CAD build for the part. Positions are in the model's coordinates, mm. Face numbers are marked on the shaded views. Coordinates: 2 decimals unless noted, no trailing zeros. Write each loop counter-clockwise with the first axis right and the second up, starting at its lowest first coordinate (ties: lowest second). Pieces come first, ordered by that corner, then holes. Notation, with made-up numbers: M -27.75,59 L -12.75,59 A26 cw -12.75,75 Z; hole C 63,55.5 d10. An arc over 180 degrees is marked long. Answer as CSV lines item,"result". Start each with the question number.
```python
from build123d import *

# Parameters (mm, degrees)
SKETCH_1_R      = 8.5
SKETCH_1_R_2    = 2.1
EXTRUDE_1_DEPTH = 6
FILLET_1_R      = 15
FILLET_2_R      = 2
SKETCH_2_R      = 2.1
EXTRUDE_2_DEPTH = 5
SKETCH_3_W      = 10
SKETCH_3_H      = 30
SKETCH_3_R      = 2.1
EXTRUDE_3_DEPTH = 7
FILLET_4_R      = 2
FILLET_5_R      = 2
CHAMFER_1_SIZE  = 1


with BuildPart() as part:
    # 草图1 → 凸台-拉伸1 (new body)
    with BuildSketch(Plane(origin=(0, 0, 0), x_dir=(1, 0, 0), z_dir=(0, 1, 0))):
        Polygon((0, 0), (100, 0), (129.781745931, -29.781745931), (158.066017178, -1.497474683), (132.13708499, 24.431457505), (70, 24.431457505), (30, 24.431457505), (-32.13708499, 24.431457505), (-58.066017178, -1.497474683), (-29.781745931, -29.781745931), align=None)
        with Locations(Location((-30.5, -5, 0), (0, 0, 270))):
            Circle(SKETCH_1_R, mode=Mode.SUBTRACT)
        with Locations(Location((130.5, -5, 0), (0, 0, 270))):
            Circle(SKETCH_1_R, mode=Mode.SUBTRACT)
        with Locations(Location((0, 10, 0), (0, 0, 270))):
            Circle(SKETCH_1_R_2, mode=Mode.SUBTRACT)
        with Locations(Location((100, 10, 0), (0, 0, 270))):
            Circle(SKETCH_1_R_2, mode=Mode.SUBTRACT)
    extrude(amount=EXTRUDE_1_DEPTH)

    # 圆角1
    fillet_1_edges = [part.edges().sort_by_distance(p)[0] for p in [
        (-29.781745931, 3, 29.781745931),
        (-58.066017178, 3, 1.497474683),
        (158.066017178, 3, 1.497474683),
        (129.781745931, 3, 29.781745931),
    ]]
    fillet(fillet_1_edges, radius=FILLET_1_R)

    # 圆角2
    fillet_2_edges = [part.edges().sort_by_distance(p)[0] for p in [
        (100, 3, 0),
        (0, 3, 0),
    ]]
    fillet(fillet_2_edges, radius=FILLET_2_R)

    # 草图2 → 凸台-拉伸2 (add)
    # profile 1 of 4: a face of its own
    with BuildSketch(Plane.XY):
        Polygon((17, 6), (23, 6), (27, 6), (27, 30), (17, 30), align=None)
        with Locations((23, 15)):
            Circle(SKETCH_2_R, mode=Mode.SUBTRACT)
        with Locations((23, 25)):
            Circle(SKETCH_2_R, mode=Mode.SUBTRACT)
    # profile 2 of 4: a face of its own
    with BuildSketch(Plane.XY):
        Polygon((27, 6), (23, 6), (17, 6), (17, 0), (27, 0), align=None)
    # profile 3 of 4: a face of its own
    with BuildSketch(Plane.XY):
        Polygon((68, 30), (68, 6), (72, 6), (78, 6), (78, 30), align=None)
        with Locations((72, 15)):
            Circle(SKETCH_2_R, mode=Mode.SUBTRACT)
        with Locations((72, 25)):
            Circle(SKETCH_2_R, mode=Mode.SUBTRACT)
    # profile 4 of 4: a face of its own
    with BuildSketch(Plane.XY):
        Polygon((72, 6), (68, 6), (68, 0), (78, 0), (78, 6), align=None)
    extrude(amount=-EXTRUDE_2_DEPTH)

    # 草图3 → 凸台-拉伸3 (add)
    # profile 1 of 2: a face of its own
    with BuildSketch(Plane(origin=(0, 30, 0), x_dir=(1, 0, 0), z_dir=(0, 1, 0))):
        with Locations((22, 15)):
            Rectangle(SKETCH_3_W, SKETCH_3_H)
        with Locations(Location((22, 25, 0), (0, 0, 270))):
            Circle(SKETCH_3_R, mode=Mode.SUBTRACT)
        with Locations(Location((22, 10, 0), (0, 0, 270))):
            Circle(SKETCH_3_R, mode=Mode.SUBTRACT)
    # profile 2 of 2: a face of its own
    with BuildSketch(Plane(origin=(0, 30, 0), x_dir=(1, 0, 0), z_dir=(0, 1, 0))):
        with Locations((73, 15)):
            Rectangle(SKETCH_3_W, SKETCH_3_H)
        with Locations(Location((73, 25, 0), (0, 0, 270))):
            Circle(SKETCH_3_R, mode=Mode.SUBTRACT)
        with Locations(Location((73, 10, 0), (0, 0, 270))):
            Circle(SKETCH_3_R, mode=Mode.SUBTRACT)
    extrude(amount=EXTRUDE_3_DEPTH)

    # 圆角4
    fillet_4_edges = [part.edges().sort_by_distance(p)[0] for p in [
        (27, 33.5, -30),
        (17, 33.5, -30),
        (78, 33.5, -30),
        (68, 33.5, -30),
    ]]
    fillet(fillet_4_edges, radius=FILLET_4_R)

    # 圆角5
    fillet_5_edges = [part.edges().sort_by_distance(p)[0] for p in [
        (-32.13708499, 3, -24.431457505),
        (132.13708499, 3, -24.431457505),
    ]]
    fillet(fillet_5_edges, radius=FILLET_5_R)

    # 倒角1
    chamfer_1_edges = [part.edges().sort_by_distance(p)[0] for p in [
        (-30.5, 0, -3.5),
        (-30.5, 6, -3.5),
        (130.5, 0, -3.5),
        (130.5, 6, -3.5),
    ]]
    chamfer(chamfer_1_edges, length=CHAMFER_1_SIZE)


solid = part.part
```
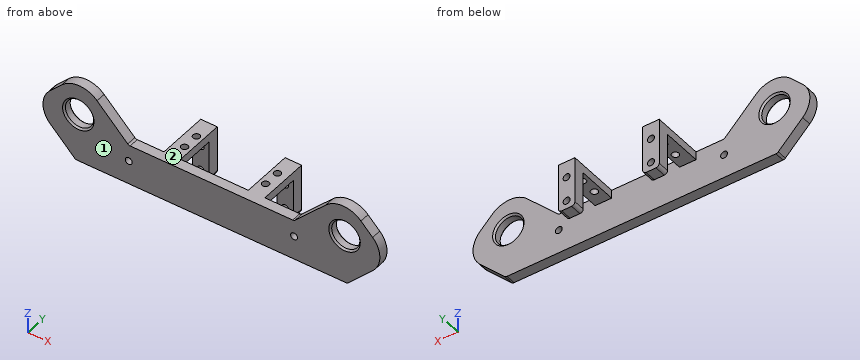
1) Pin check, flat tips, straight feed: P1, Ø6.5, axis at x = 100, z = -10, coming from the +Y side; P2, Ø3, axis at y = 5, z = -2, coming from the +X side; P3, Ø5.5, axis at x = 72, y = 15, coming from the -Z side. Stop position of each tip, or through.
2) Probe L1, parallel to Y at x = 72, z = -1.35; L2, parallel to X at y = 32, z = -10; L3, parallel to X at y = 1.8, z = -10. List the from-to ranges inside material, lowest first. Write a range as [from, to].
3) Band-saw the part on A-A, the plane y = 25. List the corners of the cut face in (x, z), plus the area to 3 significant figures.
4) Band-saw the part on C-C, the plane z = 9.5. State how many separate pieces and enclosed holes the cut face has, plus the area to 3 significant figures.
5) Two-plate mould, pull along X, no slides. Class the marked faces 1 and 2: pulls with the +X half, pulls with the -X half, needs draft (parallel to the pull), parting line crosses it, or undercut.
6) Band-saw the part on B-B, the plane x = 52. List the corners of the cut face in (y, z).
Result sheet:
1,P1,"stops at y = 6"
1,P2,"stops at x = 151.72"
1,P3,"stops at z = -5"
2,L1,"y = [0, 12.9], [17.1, 22.9], [27.1, 37]"
2,L2,"x = [17, 19.9], [24.1, 27], [68, 70.9], [75.1, 78]"
2,L3,"x = [-46.57, -2.1], [2.1, 97.9], [102.1, 146.57]"
3,outline,"M 17,-5 L 20.9,-5 L 20.9,0 L 17,0 Z; M 25.1,-5 L 27,-5 L 27,0 L 25.1,0 Z; M 68,-5 L 69.9,-5 L 69.9,0 L 68,0 Z; M 74.1,-5 L 78,-5 L 78,0 L 74.1,0 Z"
3,area,"58.0 mm²"
4,separate pieces,"4"
4,enclosed holes,"0"
4,area,"303 mm²"
5,face 1,"needs draft"
5,face 2,"undercut"
6,outline,"M 0,-24.43 L 6,-24.43 L 6,0 L 0,0 Z"
